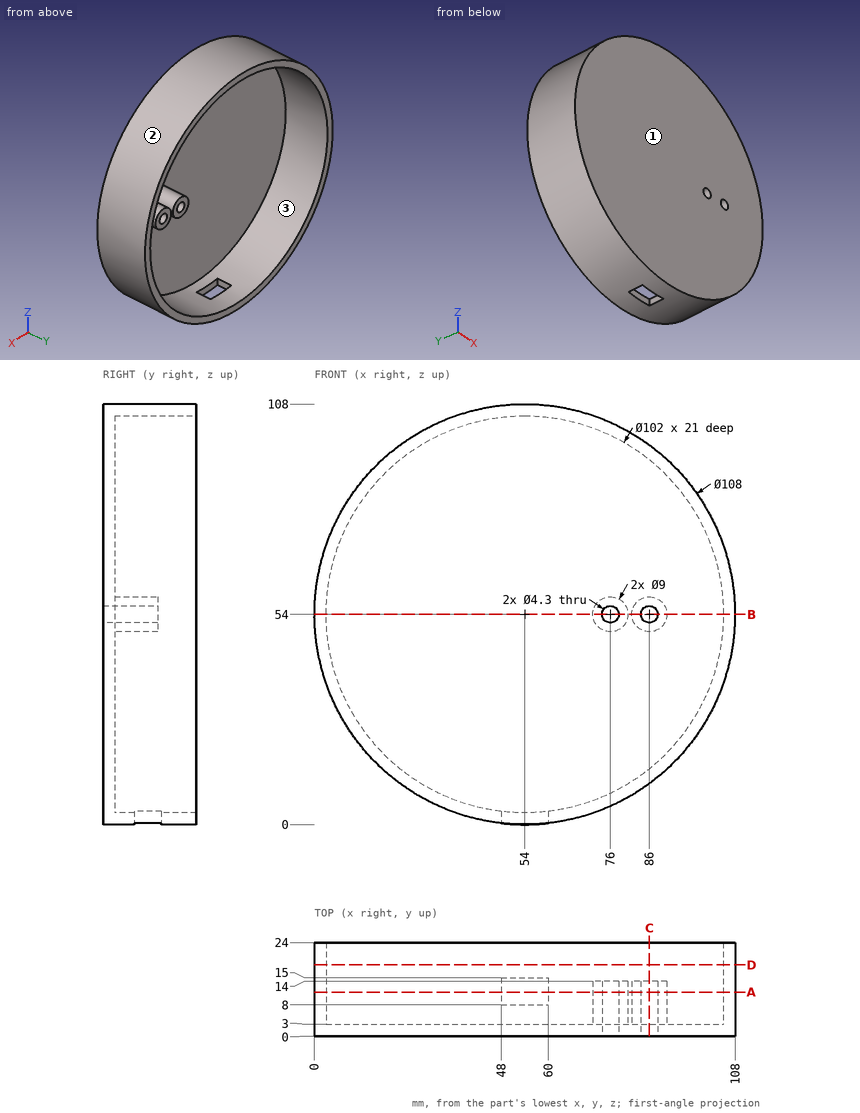
Verification items for this drawing (mm, ordinates from the low corner). Give positions to 0.01 mm unless a question says otherwise; leave off trailing zeros. Loops run counter-clockwise (first coordinate to the right, second up) from the corner with the lowest first, then second, coordinate; pieces in that order, holes last. Notation, with made-up numbers: (61.25, 78.5) - (75.25, 78.5) arc R33 ccw to (75.25, 114.5) - close; hole circle Ø2 at (-12, 64.25). An arc over 180 degrees is marked (long way). Write item = value, one per line. Start each with the question number.
Q1. Mould release check, pull along X, two halves, no side actions. Record for the marked faces 1, 2 and 3: released by +X, released by -X, zero draft, split by the parting line, or undercut.
Q2. Thickness scan on line 1 (X direction, y = 6.5, z = 54); line 2 (Z direction, x = 54, y = 7.75); line 3 (Z direction, x = 76, y = 3.5). Record the ranges inside material, lowest first.
Q3. Cross-section at A-A, the plane y = 11.25. Enter the section's corners in (x, z), and give its area (3 significant figures).
Q4. Cross-section at C-C, the plane x = 86. Enter the section's corners in (y, z).
Q5. Depth check by flat-ended pin: P1, Ø1, axis at x = 70.5, z = 60, coming from the -Y side; P2, Ø6, axis at y = 13, z = 15, coming from the +X side; P3, Ø8, axis at y = 16, z = 49.5, coming from the +X side; P4, Ø4, axis at x = 76, z = 54, coming from the +Y side. Enter the tip coordinate at first touch or a pass-through.
Q6. Cross-section at B-B, the plane z = 54. Enter the section's corners in (x, y), and give its area (3 significant figures).
Q7. Cross-section at D-D, the plane y = 18.25. Enter the section's corners in (x, z), and give its area (3 significant figures).
Answer key:
q1.face_1 = zero draft
q1.face_2 = split by the parting line
q1.face_3 = undercut
q2.line_1 = 0 to 3, 71.5 to 73.85, 78.15 to 80.5, 81.5 to 83.85, 88.15 to 90.5, 105 to 108
q2.line_2 = 0 to 3, 105 to 108
q2.line_3 = 4.68 to 7.99, 49.5 to 51.85, 56.15 to 58.5, 100.01 to 103.32
q3.outline = (48, 0.33) - (48, 3.35) arc R51 cw (long way) to (60, 3.35) - (60, 0.33) arc R54 ccw (long way) to start; circle Ø9 at (76, 54); circle Ø9 at (86, 54); hole circle Ø4.3 at (76, 54); hole circle Ø4.3 at (86, 54)
q3.area = 1,050 mm^2
q4.outline = (0, 10.5) - (24, 10.5) - (24, 14.29) - (3, 14.29) - (3, 49.5) - (14, 49.5) - (14, 51.85) - (0, 51.85) - close; (0, 56.15) - (14, 56.15) - (14, 58.5) - (3, 58.5) - (3, 93.71) - (24, 93.71) - (24, 97.5) - (0, 97.5) - close
q5.P1 = 0
q5.P2 = 94.25
q5.P3 = 108
q5.P4 = through
q6.outline = (0, 0) - (73.85, 0) - (73.85, 14) - (71.5, 14) - (71.5, 3) - (3, 3) - (3, 24) - (0, 24) - close; (78.15, 0) - (83.85, 0) - (83.85, 14) - (81.5, 14) - (81.5, 3) - (80.5, 3) - (80.5, 14) - (78.15, 14) - close; (88.15, 0) - (108, 0) - (108, 24) - (105, 24) - (105, 3) - (90.5, 3) - (90.5, 14) - (88.15, 14) - close
q6.area = 528 mm^2
q7.outline = circle Ø108 at (54, 54); hole circle Ø102 at (54, 54)
q7.area = 990 mm^2
